Could you check a few things on this model? Use its own coordinates, in mm. A direction names the side the tool comes from. Coordinates: 2 decimals unless noted, no trailing zeros. Order: outer loops, then holes, each group sorted by start corner. A loop starts at its lowest first (then second) coordinate and runs counter-clockwise, first axis right, second up.
```python
from build123d import *

# Parameters (mm, degrees)
SKETCH_R          = 19.5
PAD_DEPTH         = 20
SKETCH002_R       = 2
POCKET_DEPTH      = 21
POCKET_DEPTH_BACK = -21


with BuildPart() as part:
    # Sketch → Pad (new body)
    with BuildSketch(Plane.XY):
        Circle(SKETCH_R)
        with BuildLine():
            ThreePointArc((14.5, 7.874008), (0, 16.5), (-14.5, 7.874008))
            Line((-14.5, 7.874008), (-14.5, -7.874008))
            ThreePointArc((-14.5, -7.874008), (0, -16.5), (14.5, -7.874008))
            Line((14.5, 7.874008), (14.5, -7.874008))
        make_face(mode=Mode.SUBTRACT)
    extrude(amount=PAD_DEPTH)

    # Sketch001 → Revolution (revolve)
    with BuildSketch(Plane.XZ):
        Polygon((-19.5, 20), (-18, 21.5), (-16.5, 20), align=None)
    revolve(axis=Axis((0, 0, 0), (0, 0, 1)))

    # Sketch002 → Pocket (cut, two sides)
    with BuildSketch(Plane.YZ) as pocket_sk:
        with Locations((0, 8)):
            Circle(SKETCH002_R)
    extrude(amount=-POCKET_DEPTH, mode=Mode.SUBTRACT)
    extrude(pocket_sk.sketch, amount=-POCKET_DEPTH_BACK, mode=Mode.SUBTRACT)


solid = part.part
```
Item 1: Suppose I cut it at C-C (z = 8.5). List the corners of the cut face in (x, y) for me.
Item 2: Suppose I cut it at A-A (y = 0). List the corners of the cut face in (x, z) for me.
Item 3: Suppose I cut it at B-B (z = 18.5). List the corners of the cut face in (x, y) for me, and give its area (3 significant figures).
Item 4: For pin 1 Ø1 at (y, z) = (-12, 3.5) entering from -X; pin 2 Ø4 at (y, z) = (14.5, 2) entering from -X; pin 3 Ø10 at (y, z) = (13, 19) entering from -X, each with a flat end and sliding along its axis, tell me the tip position at first contact or that it passes through.
Item 5: Thinking about a two-plate mould opening in Y: for faces 1 (the face through (14.5, 2, 10)), 2 (the face through (-15, 2, 0)), 3 (the face through (18.6, 5.86, 9.86)), which applies, +Y half, -Y half, draft (parallel to the pull), parting line (faces both ways), or undercut?
Item 6: I need wall thicknesses on line 1 (Y direction, x = -2.5, z = 12.25); line 2 (X direction, y = -5, z = 3); line 3 (Z direction, x = 17, y = 0). Which ranges of each line are inside material? Lowest first, please.
Item 7: Which directions (+Z, -Z, +X, -X, +Y, -Y) give clear straight access to the entire face, cutting with the end or side of a thin tool? Please do faces 4 (the face through (17, 0, 10)), 5 (the face through (15, 0, 20)), 6 (the face through (-0.2, -16.5, 9.9)).
Geometry results:
1. outline: (-19.4, -1.94) arc R19.5 ccw to (19.4, -1.94) - (14.5, -1.94) - (14.5, -7.87) arc R16.5 cw to (-14.5, -7.87) - (-14.5, -1.94) - close; (-19.4, 1.94) - (-14.5, 1.94) - (-14.5, 7.87) arc R16.5 cw to (14.5, 7.87) - (14.5, 1.94) - (19.4, 1.94) arc R19.5 ccw to start
2. outline: (-19.5, 0) - (-14.5, 0) - (-14.5, 6) - (-19.5, 6) - close; (-19.5, 10) - (-14.5, 10) - (-14.5, 20) - (-16.5, 20) - (-18, 21.5) - (-19.5, 20) - close; (14.5, 0) - (19.5, 0) - (19.5, 6) - (14.5, 6) - close; (14.5, 10) - (19.5, 10) - (19.5, 20) - (18, 21.5) - (16.5, 20) - (14.5, 20) - close
3. outline: circle Ø39 at (0, 0); hole (-14.5, -7.87) arc R16.5 ccw to (14.5, -7.87) - (14.5, 7.87) arc R16.5 ccw to (-14.5, 7.87) - close
3. area: 382 mm2
4. pin 1: stops at x = -15.75
4. pin 2: stops at x = -14.97
4. pin 3: stops at x = -17.78
5. face 1: undercut
5. face 2: draft
5. face 3: parting line
6. line 1: y = -19.34 to -16.31, 16.31 to 19.34
6. line 2: x = -18.85 to -14.5, 14.5 to 18.85
6. line 3: z = 0 to 6, 10 to 20.5
7. face 4: +X, -X
7. face 5: +Z
7. face 6: +Z, -Z
